Can you work these out from the model? Positions are in its coordinate system, mm. Give positions to 0.01 mm unless a question says otherwise; leave off trailing zeros. Order: outer loops, then holes, each group sorted by start corner. A loop starts at its lowest first (then second) coordinate and runs counter-clockwise, first axis right, second up.
Item 1: I want a section at A-A, the plane x = 218. Write out the boundary of the cut face in (y, z).
Item 2: I want a section at B-B, the plane y = 11.5. Count the separate pieces of the cut face and the enclosed holes in it, then the cut area to 3 significant figures.
Item 3: If we mould it in two halves opening along Z, with no side actions, what happens to faces 1 (the flat face through (4, 17.78, 3)), 2 (the flat face through (-4, 9, -228.6)), 3 (the cylindrical face through (-76.455, 8.766, 81.278))? For each: +Z half, -Z half, draft (parallel to the pull), parting line (faces both ways), or undercut.
Item 4: If I drill on line 1 along Z through (x, y) = (192.5, 14); line 2 along X through (y, z) = (7, -180); line 3 along X through (y, z) = (15, 153), over which ranges is the centre line in solid material (lowest first)?
Autodesk Inventor part; units mm, degrees
ref_plane "YZ Plane" through (0, 0, 0) normal (1, 0, 0) x (0, 1, 0)
ref_plane "XZ Plane" through (0, 0, 0) normal (0, 1, 0) x (-1, 0, 0)
ref_plane "XY Plane" through (0, 0, 0) normal (0, 0, 1) x (1, 0, 0)
sketch "Sketch1" plane through (0, 0, 0) normal (0, 1, 0) x (-1, 0, 0)
  line L0 (-304.8, 228.6) -> (304.8, 228.6)
  line L1 (304.8, 228.6) -> (304.8, -228.6)
  line L2 (304.8, -228.6) -> (-304.8, -228.6)
  line L3 (-304.8, -228.6) -> (-304.8, 228.6)
  line L4 (-304.8, 228.6) -> (304.8, -228.6) construction
  line L5 (304.8, 228.6) -> (-304.8, -228.6) construction
  line L6 (-304.8, 228.6) -> (304.8, 228.6)
  line L7 (304.8, 228.6) -> (304.8, -228.6)
  line L8 (304.8, -228.6) -> (-304.8, -228.6)
  line L9 (-304.8, -228.6) -> (-304.8, 228.6)
  line L10 (-304.8, 228.6) -> (304.8, -228.6) construction
  line L11 (304.8, 228.6) -> (-304.8, -228.6) construction
  point P0 (0, 0)
  point P1 (0, 0)
  dimension "d0" = 609.6
  dimension "d1" = 457.2
  dimension "d4" = 609.6
  dimension "d5" = 457.2
sketch "Sketch2" plane through (0, 0, 0) normal (0, 1, 0) x (-1, 0, 0)
  line L0 (-304.8, 228.6) -> (304.8, 228.6)
  line L1 (304.8, 228.6) -> (304.8, -228.6)
  line L2 (304.8, -228.6) -> (-304.8, -228.6)
  line L3 (-304.8, -228.6) -> (-304.8, 228.6)
  line L4 (-304.8, 228.6) -> (304.8, -228.6) construction
  line L5 (304.8, 228.6) -> (-304.8, -228.6) construction
  circle A0 centre (228.8418, 180.9093) radius 3.175
  circle A1 centre (151.3083, 180.9093) radius 3.175
  circle A2 centre (112.5416, 113.7633) radius 3.175
  circle A3 centre (151.3083, 46.6174) radius 3.175
  circle A4 centre (228.8418, 46.6174) radius 3.175
  circle A5 centre (267.6086, 113.7633) radius 3.175
  circle A6 centre (190.0751, 113.7633) radius 51.1302
  line L6 (-304.8, 228.6) -> (304.8, 228.6)
  line L7 (304.8, 228.6) -> (304.8, -228.6)
  line L8 (304.8, -228.6) -> (-304.8, -228.6)
  line L9 (-304.8, -228.6) -> (-304.8, 228.6)
  line L10 (-304.8, 228.6) -> (304.8, -228.6) construction
  line L11 (304.8, 228.6) -> (-304.8, -228.6) construction
  circle A7 centre (228.8418, 180.9093) radius 3.175
  circle A8 centre (151.3083, 180.9093) radius 3.175
  circle A9 centre (112.5416, 113.7633) radius 3.175
  circle A10 centre (151.3083, 46.6174) radius 3.175
  circle A11 centre (228.8418, 46.6174) radius 3.175
  circle A12 centre (267.6086, 113.7633) radius 3.175
  circle A13 centre (190.0751, 113.7633) radius 51.1302
  point P0 (0, 0)
  point P1 (0, 0)
  point P2 (0, 0)
  dimension "d6" = 609.6
  dimension "d7" = 457.2
  dimension "d8" = 609.6
  dimension "d9" = 457.2
extrude "Extrusion1" add sketch "Sketch1" along normal blind 17.78
sketch "Sketch3" plane through (0, 17.78, 0) normal (0, 1, 0) x (1, 0, 0)
  circle A0 centre (-190.0751, -113.7633) radius 51.1302
  circle A1 centre (-151.3083, -46.6174) radius 3.175
  circle A2 centre (-112.5416, -113.7633) radius 3.175
  circle A3 centre (-151.3083, -180.9093) radius 3.175
  circle A4 centre (-228.8418, -180.9093) radius 3.175
  circle A5 centre (-267.6086, -113.7633) radius 3.175
  circle A6 centre (-228.8418, -46.6174) radius 3.175
  point P0 (0, 0)
hole "Hole1" at (-228.8418, 17.78, 180.9093) at (-267.6086, 17.78, 113.7633) at (-228.8418, 17.78, 46.6174) at (-151.3083, 17.78, 46.6174) at (-112.5416, 17.78, 113.7633) at (-151.3083, 17.78, 180.9093) direction (0, -1, 0) diameter 6.35 end through all
hole "Hole2" at (-190.0751, 0, 113.7633) direction (0, 1, 0) diameter 101.6 depth 46.0375
mirror "Mirror1" about plane through (0, 0, 0) normal (1, 0, 0) of "Hole1", "Hole2"
mirror "Mirror2" about plane through (0, 0, 0) normal (0, 0, 1) of "Hole1", "Hole2", "Mirror1"
sketch "Sketch5" plane through (0, 17.78, 0) normal (0, 1, 0) x (1, 0, 0)
  line L0 (0, 0) -> (82.6543, 82.6543) construction
  line L1 (0, 0) -> (116.8908, 0) construction
  line L2 (0, 0) -> (-82.6543, 82.6543) construction
  line L3 (0, 0) -> (-82.6543, -82.6543) construction
  line L4 (0, 0) -> (116.8908, 0) construction
  line L5 (0, 0) -> (82.6543, -82.6543) construction
  line L6 (0, 0) -> (116.8908, 0) construction
  circle A0 centre (82.6543, 82.6543) radius 6.35
  circle A1 centre (-82.6543, 82.6543) radius 6.35
  circle A2 centre (-82.6543, -82.6543) radius 6.35
  circle A3 centre (82.6543, -82.6543) radius 6.35
  dimension "d41" = 116.8908
  dimension "d42" = 45
  dimension "d43" = 116.8908
  dimension "d44" = 116.8908
  dimension "d45" = 135
  dimension "d46" = 116.8908
  dimension "d47" = 45
  dimension "d48" = 12.7
  dimension "d49" = 12.7
  dimension "d50" = 12.7
  dimension "d51" = 12.7
hole "Hole4" at (82.6543, 17.78, -82.6543) at (82.6543, 17.78, 82.6543) at (-82.6543, 17.78, 82.6543) at (-82.6543, 17.78, -82.6543) direction (0, -1, 0) diameter 12.7 end through all
properties part number "sheetmappingv5"
Results list:
1. outline: (0, -228.6) - (17.78, -228.6) - (17.78, -156.2) - (0, -156.2) - close; (0, -71.33) - (17.78, -71.33) - (17.78, 71.33) - (0, 71.33) - close; (0, 156.2) - (17.78, 156.2) - (17.78, 228.6) - (0, 228.6) - close
2. separate pieces: 1
2. enclosed holes: 32
2. area: 245,000 mm2
3. face 1: draft
3. face 2: -Z half
3. face 3: undercut
4. line 1: z = -228.6 to -164.51, -63.02 to 63.02, 164.51 to 228.6
4. line 2: x = -304.8 to -231.88, -225.8 to -154.35, -148.27 to 148.27, 154.35 to 225.8, 231.88 to 304.8
4. line 3: x = -304.8 to -222.34, -157.81 to 157.81, 222.34 to 304.8
